For this review, use the dimensioned drawing (mm, ordinates from the lowest corner) and the shaded views. Round coordinates to 2 decimals unless told otherwise and drop trailing zeros. Write each loop counter-clockwise with the first axis right and the second up, starting at its lowest first coordinate (ties: lowest second). Pieces come first, ordered by that corner, then holes. Notation, with made-up numbers: M 51,48 L 95,48 A37 cw 95,84 Z; hole C 51,14 d9. An arc over 180 degrees is marked long. One line per question, with ' | ' between items. Start each with the question number.
Item 1: Add section B-B, the plane y = 6.5. State the section outline as (x, z) points (3 decimals).
Item 2: Add section A-A, the plane x = 5. State the section outline as (y, z) points (3 decimals).
Item 3: Draft analysis for pull direction Y (two halves, no side actions). For the marked faces 1, 2 and 3, state which applies: released by +Y, released by -Y, zero draft, split by the parting line, or undercut.
Item 4: Insertion check: pin 1 Ø2.5 at (x, y) = (11, 21.5) entering from +Z. The pin has a flat end and moves straight along its axis. Give the tip position at first contact, or say it passes through.
Item 5: Add section D-D, the plane z = 1. Give the number of separate pieces and of enclosed holes in the cut face, and give its area (3 significant figures).
Item 6: For L1, parallel to Y at x = 5, z = 3 (3 decimals); L2, parallel to Y at x = 2, z = 2.25 (3 decimals); L3, parallel to Y at x = 11.5, z = 4.5, list the stretches that pass through material, from the lowest coordinate up.
Item 7: Add section C-C, the plane x = 14. State the section outline as (y, z) points (3 decimals).
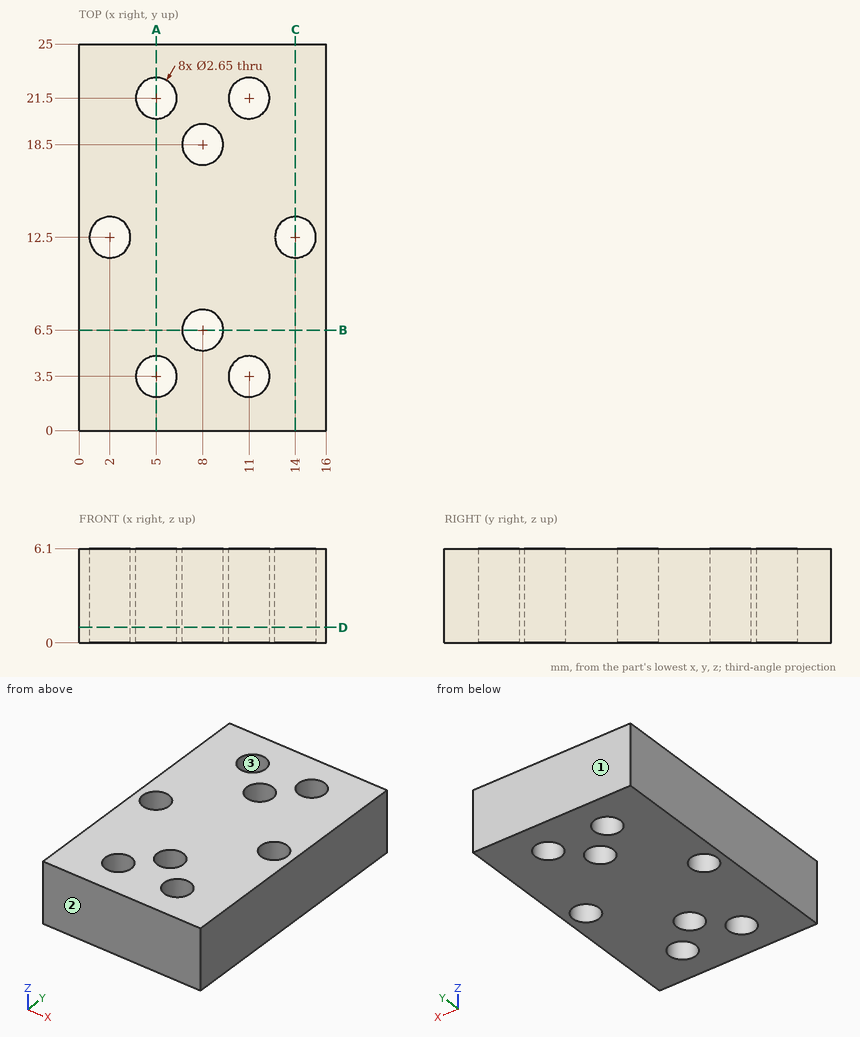
Computed values:
1) outline: M 0,0 L 6.675,0 L 6.675,6.1 L 0,6.1 Z; M 9.325,0 L 16,0 L 16,6.1 L 9.325,6.1 Z
2) outline: M 0,0 L 2.175,0 L 2.175,6.1 L 0,6.1 Z; M 4.825,0 L 20.175,0 L 20.175,6.1 L 4.825,6.1 Z; M 22.825,0 L 25,0 L 25,6.1 L 22.825,6.1 Z
3) face 1: released by +Y | face 2: released by -Y | face 3: undercut
4) pin 1: passes through
5) separate pieces: 1 | enclosed holes: 8 | area: 356 mm^2
6) L1: y = 0 to 2.175, 4.825 to 20.175, 22.825 to 25 | L2: y = 0 to 11.175, 13.825 to 25 | L3: y = 0 to 2.27, 4.73 to 20.27, 22.73 to 25
7) outline: M 0,0 L 11.175,0 L 11.175,6.1 L 0,6.1 Z; M 13.825,0 L 25,0 L 25,6.1 L 13.825,6.1 Z
